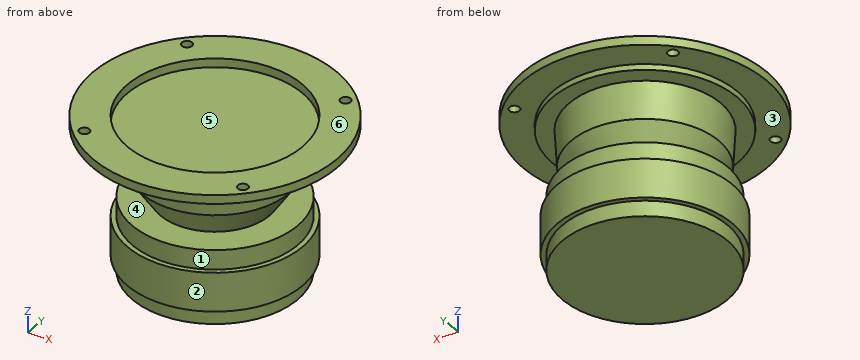
```python
from build123d import *

# Parameters (mm, degrees)
F0_W     = 42.5
F0_H     = 8
F1_R     = 62.75
F1_R_2   = 2.6
F1_R_3   = 45
F3_DEPTH = 4.5


with BuildPart() as f2:
    # F0 (on Right) → F2 (revolve)
    with BuildSketch(Plane.YZ):
        Polygon((0, -37), (0, 0), (-47.5, 0), (-47.5, -3), (-39, -3), (-38, -22), (-28, -37), align=None)
        Polygon((0, -47), (0, -37), (-28, -37), (-42.5, -37), (-42.5, -47), align=None)
        Polygon((0, -67), (0, -47), (-42.5, -47), (-45, -47), (-45, -67), (-42.5, -67), align=None)
        with Locations((-21.25, -71)):
            Rectangle(F0_W, F0_H)
    revolve(axis=Axis((0, 0, -38.677778095), (0, 0, -1)))

    # F1 (on Top) → F3 (join)
    with BuildSketch(Plane.XY):
        Circle(F1_R)
        with Locations((-40.6586399182, -40.6586399182)):
            Circle(F1_R_2, mode=Mode.SUBTRACT)
        with Locations((40.6586399182, -40.6586399182)):
            Circle(F1_R_2, mode=Mode.SUBTRACT)
        with Locations((-40.6586399182, 40.6586399182)):
            Circle(F1_R_2, mode=Mode.SUBTRACT)
        Circle(F1_R_3, mode=Mode.SUBTRACT)
        with Locations((40.6586399182, 40.6586399182)):
            Circle(F1_R_2, mode=Mode.SUBTRACT)
    extrude(amount=F3_DEPTH)


solid = f2.part
```
CAD build for the part. Positions are in the model's coordinates, mm. Face numbers are marked on the shaded views. A direction names the side the tool comes from. Round coordinates to 2 decimals unless told otherwise and drop trailing zeros. Order: outer loops, then holes, each group sorted by start corner. A loop starts at its lowest first (then second) coordinate and runs counter-clockwise, first axis right, second up. Notation, with made-up numbers: (84, 57.5) -> (112, 57.5) arc R14 cw to (112, 68.5) -> close; hole circle Ø2 at (69, 47.5). An arc over 180 degrees is marked (long way). One line per question, with ' | ' between items.
Q1. Two-plate mould, pull along Z, no slides. Class the marked faces 1, 2 and 3: released by +Z, released by -Z, zero draft, split by the parting line, or undercut.
Completed:
face 1: undercut | face 2: zero draft | face 3: released by -Z
Q2. Which spindle directions (+Z, -Z, +X, -X, +Y, -Y) get a long thin tool onto all of the face, cutting with end or side? Do the marked faces 4, 5 and 6. Say none if no direction does.
Completed:
face 4: none | face 5: +Z | face 6: +Z, +X, -X, +Y, -Y
Q3. Drop flat-ended pins along their axis: pin 1 (3 mm diameter, centred on x = -11.5, y = -1, fed in from +Z); pin 2 (8 mm diameter, centred on y = 20, z = -67, fed in from -X); pin 3 (12 mm diameter, centred on y = -24, z = -9.5, fed in from -X). Give the stop position or say it passes through.
Completed:
pin 1: stops at z = 0 | pin 2: stops at x = -42.06 | pin 3: stops at x = -34.23
Q4. Slice it at C-C (z = -62). Write the cut outline in (x, y), then the cut area to 3 significant figures.
Completed:
outline: circle Ø90 at (0, 0) | area: 6,360 mm^2
Q5. Slice it at D-D (z = -29.5). Write the cut outline in (x, y).
Completed:
outline: circle Ø66 at (0, 0)
Q6. Probe probe 1 along Z at (x, y) = (-13, 20.5); probe 2 along Z at (x, y) = (-27, 55); probe 3 along Z at (x, y) = (-36, -20). List the from-to ranges inside material, lowest first.
Completed:
probe 1: z = -75 to 0 | probe 2: z = 0 to 4.5 | probe 3: z = -75 to -37, -3 to 0
